```python
from build123d import *

# Parameters (mm, degrees)
SKETCH1_W                                           = 28
SKETCH1_H                                           = 84
BOSS_EXTRUDE2_DEPTH                                 = 15
SKETCH7_W                                           = 54
SKETCH7_H                                           = 12
CUT_EXTRUDE2_DEPTH                                  = 1
CUT_EXTRUDE2_DEPTH_BACK                             = 29
SKETCH6_W                                           = 20
SKETCH6_H                                           = 40.4
CUT_EXTRUDE1_DEPTH                                  = 16
SKETCH8_W                                           = 28
SKETCH8_H                                           = 5
CUT_EXTRUDE3_DEPTH                                  = 7
SKETCH9_R                                           = 1.45
CUT_EXTRUDE4_DEPTH                                  = 6
SKETCH11_R                                          = 4
CUT_EXTRUDE5_DEPTH                                  = 1
CUT_EXTRUDE5_DEPTH_BACK                             = 29
SKETCH12_R                                          = 1.5
CUT_EXTRUDE6_DEPTH                                  = 8
SKETCH13_R                                          = 1.5
CUT_EXTRUDE7_DEPTH                                  = 16
BOSS_EXTRUDE3_DEPTH                                 = 20
CUT_EXTRUDE10_DEPTH                                 = 25
CBORE_FOR_M3_HEX_SOCKET_HEAD_CAP_SCREW1_D           = 3.2
CBORE_FOR_M3_HEX_SOCKET_HEAD_CAP_SCREW1_CBORE_D     = 6.5
CBORE_FOR_M3_HEX_SOCKET_HEAD_CAP_SCREW1_CBORE_DEPTH = 3.4


with BuildPart() as part:
    # Sketch1 → Boss-Extrude2 (new body)
    with BuildSketch(Plane(origin=(0, 0, 0), x_dir=(1, 0, 0), z_dir=(0, 1, 0))):
        with Locations((14, 42)):
            Rectangle(SKETCH1_W, SKETCH1_H)
    extrude(amount=BOSS_EXTRUDE2_DEPTH)

    # Sketch7 → Cut-Extrude2 (cut, two sides)
    with BuildSketch(Plane(origin=(28, 0, 0), x_dir=(0, 0, -1), z_dir=(1, 0, 0))) as cut_extrude2_sk:
        with Locations((42, 6)):
            Rectangle(SKETCH7_W, SKETCH7_H)
    extrude(amount=CUT_EXTRUDE2_DEPTH, mode=Mode.SUBTRACT)
    extrude(cut_extrude2_sk.sketch, amount=-CUT_EXTRUDE2_DEPTH_BACK, mode=Mode.SUBTRACT)

    # Sketch6 → Cut-Extrude1 (cut, through all)
    with BuildSketch(Plane(origin=(0, 15, 0), x_dir=(1, 0, 0), z_dir=(0, 1, 0))):
        with Locations((14, 38.2)):
            Rectangle(SKETCH6_W, SKETCH6_H)
    extrude(amount=-CUT_EXTRUDE1_DEPTH, mode=Mode.SUBTRACT)

    # Sketch8 → Cut-Extrude3 (cut)
    with BuildSketch(Plane.XY):
        with Locations((14, 9.5)):
            Rectangle(SKETCH8_W, SKETCH8_H)
    extrude(amount=-CUT_EXTRUDE3_DEPTH, mode=Mode.SUBTRACT)

    # Sketch9 → Cut-Extrude4 (cut)
    with BuildSketch(Plane(origin=(0, 15, 0), x_dir=(1, 0, 0), z_dir=(0, 1, 0))):
        with Locations((7.5, 13.5)):
            Circle(SKETCH9_R)
        with Locations((20.5, 13.5)):
            Circle(SKETCH9_R)
        with Locations((7.5, 62.9)):
            Circle(SKETCH9_R)
        with Locations((20.5, 62.9)):
            Circle(SKETCH9_R)
    extrude(amount=-CUT_EXTRUDE4_DEPTH, mode=Mode.SUBTRACT)

    # Sketch11 → Cut-Extrude5 (cut, two sides)
    with BuildSketch(Plane.ZY) as cut_extrude5_sk:
        with Locations((-10, 1.5)):
            Circle(SKETCH11_R)
        with Locations((-74, 1.5)):
            Circle(SKETCH11_R)
    extrude(amount=CUT_EXTRUDE5_DEPTH, mode=Mode.SUBTRACT)
    extrude(cut_extrude5_sk.sketch, amount=-CUT_EXTRUDE5_DEPTH_BACK, mode=Mode.SUBTRACT)

    # Sketch12 → Cut-Extrude6 (cut)
    with BuildSketch(Plane.XZ):
        with Locations((4, -3.5)):
            Circle(SKETCH12_R)
        with Locations((24, -3.5)):
            Circle(SKETCH12_R)
    extrude(amount=-CUT_EXTRUDE6_DEPTH, mode=Mode.SUBTRACT)

    # Sketch13 → Cut-Extrude7 (cut, through all)
    with BuildSketch(Plane.XZ):
        with Locations((4, -80.5)):
            Circle(SKETCH13_R)
        with Locations((24, -80.5)):
            Circle(SKETCH13_R)
    extrude(amount=-CUT_EXTRUDE7_DEPTH, mode=Mode.SUBTRACT)

    # Sketch15 → Boss-Extrude3 (add)
    with BuildSketch(Plane(origin=(0, 0, -84), x_dir=(-1, 0, 0), z_dir=(0, 0, -1))):
        with BuildLine():
            Line((-28, 15), (0, 15))
            Line((0, 15), (0, 8.75))
            Line((0, 8.75), (-10.200328962, 8.75))
            ThreePointArc((-10.200328962, 8.75), (-15.594420664, 11.168490527), (-17.506165925, 5.574694698))
            Line((-17.506165925, 5.574694698), (-10.466462197, 5.625403884))
            ThreePointArc((-10.466462197, 5.625403884), (-10.271009725, 6.05271581), (-10.127016654, 6.5))
            Line((-10.127016654, 6.5), (0, 6.5))
            Line((0, 6.5), (0, 0))
            Line((0, 0), (-28, 0))
            Line((-28, 0), (-28, 15))
        make_face()
    extrude(amount=BOSS_EXTRUDE3_DEPTH)

    # Sketch17 → Cut-Extrude10 (cut)
    with BuildSketch(Plane(origin=(0, 0, -104), x_dir=(-1, 0, 0), z_dir=(0, 0, -1))):
        with BuildLine():
            Line((0, 8.75), (-10.200328962, 8.75))
            ThreePointArc((-10.200328962, 8.75), (-15.594420664, 11.168490527), (-17.506165925, 5.574694698))
            Line((-17.506165925, 5.574694698), (-10.466462197, 5.625403884))
            ThreePointArc((-10.466462197, 5.625403884), (-10.271009725, 6.05271581), (-10.127016654, 6.5))
            Line((-10.127016654, 6.5), (0, 6.5))
            Line((0, 6.5), (0, 8.75))
        make_face()
    extrude(amount=-CUT_EXTRUDE10_DEPTH, mode=Mode.SUBTRACT)

    # CBORE for M3 Hex Socket Head Cap Screw1 (through all)
    with Locations(Plane(origin=(7.226315369, 0, -88), x_dir=(0, 0, -1), z_dir=(0, -1, 0))):
        with Locations((0, 0), (10, 0)):
            CounterBoreHole(CBORE_FOR_M3_HEX_SOCKET_HEAD_CAP_SCREW1_D / 2, CBORE_FOR_M3_HEX_SOCKET_HEAD_CAP_SCREW1_CBORE_D / 2, CBORE_FOR_M3_HEX_SOCKET_HEAD_CAP_SCREW1_CBORE_DEPTH)


solid = part.part
```
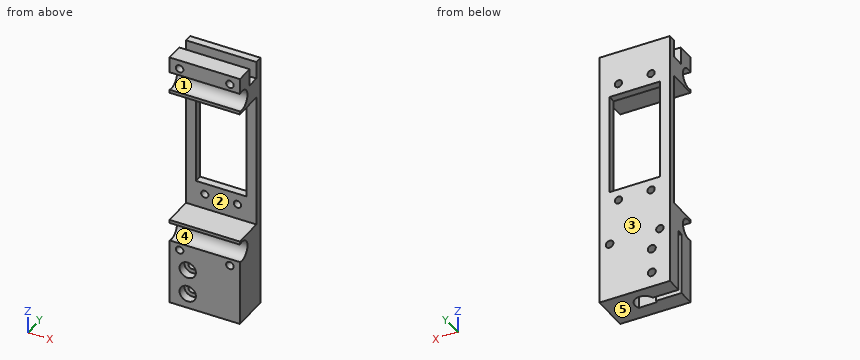
The model under review builds one solid part; all positions refer to its coordinate system, in mm. Face numbers are marked on the shaded views. A direction names the side the tool comes from. Coordinates: 2 decimals unless noted, no trailing zeros. Write each loop counter-clockwise with the first axis right and the second up, starting at its lowest first coordinate (ties: lowest second). Pieces come first, ordered by that corner, then holes. Notation, with made-up numbers: (72.25, -6) -> (121.25, -6) arc R12 ccw to (121.25, 15) -> close; hole circle Ø11 at (59.25, 35.5). An arc over 180 degrees is marked (long way). One line per item, written item: value. Start each with the question number.
Q1. Add section A-A, the plane y = 1. Count the separate pieces of the cut face and the enclosed holes in it, then the cut area to 3 significant figures.
Q2. For the marked faces 1 and 2, list the 3-axis set-ups (+Z, -Z, +X, -X, +Y, -Y) from which the entire face can be reached by the end or side of a thin tool; tool diameter is ignored.
Q3. Add section C-C, the plane x = 20.5. Give the boundary of the cut face in (y, z), then the cut area to 3 significant figures.
Q4. The part is to be moulded in two halves that separate along Z. For the marked faces 3, 4 and 5, say which applies: +Z half, -Z half, draft (parallel to the pull), parting line (faces both ways), or undercut.
Q5. Clearance check with flat-ended pins moving along their axes: P1, Ø5, axis at x = 7, z = -98, coming from the -Y side; P2, Ø1.7, axis at x = 7.5, z = -13.5, coming from the +Y side; P3, Ø3.5, axis at x = 20.5, z = -13.5, coming from the -Y side; P4, Ø12, axis at x = 3.5, z = -54, coming from the -Y side. State where each tip first meets the part, or that it passes through.
Q6. To check wall thickness, follow probe 1 along X at (y, z) = (10.8, -13.5); probe 2 along Z at (x, y) = (17.25, 1.5); probe 3 along Z at (x, y) = (20.5, 13.2). State the ranges of each line that lie inside material, in increasing order.
Q7. Add section D-D, the plane x = 14. Give the boundary of the cut face in (y, z).
Q8. Add section B-B, the plane z = -62.9. Give the boundary of the cut face in (x, y).
Response:
1. separate pieces: 4
1. enclosed holes: 6
1. area: 861 mm²
2. face 1: +X, -X
2. face 2: +X, -X, -Y
3. outline: (0, -104) -> (15, -104) -> (15, -64.35) -> (12, -64.35) -> (12, -69) -> (0, -69) -> (0, -70.29) arc R4 cw (long way) to (0, -77.71) -> close; (0, -15) -> (12, -15) -> (12, -18) -> (15, -18) -> (15, -14.95) -> (9, -14.95) -> (9, -12.05) -> (15, -12.05) -> (15, 0) -> (12, 0) -> (12, -7) -> (7, -7) -> (7, 0) -> (0, 0) -> (0, -6.29) arc R4 cw (long way) to (0, -13.71) -> close; (12, -61.45) -> (15, -61.45) -> (15, -58.4) -> (12, -58.4) -> close
3. area: 656 mm²
4. face 3: draft
4. face 4: undercut
4. face 5: -Z half
5. P1: y = 3.4
5. P2: y = 9
5. P3: y = 0
5. P4: y = 12
6. probe 1: 0 to 6.05, 8.95 to 19.05, 21.95 to 28
6. probe 2: -104 to -78, -70 to -69, -15 to -14, -6 to 0
6. probe 3: -104 to -64.35, -61.45 to -58.4, -18 to -14.95, -12.05 to 0
7. outline: (0, -104) -> (5.6, -104) -> (5.6, -79) -> (11.5, -79) -> (11.5, -104) -> (15, -104) -> (15, -58.4) -> (12, -58.4) -> (12, -69) -> (0, -69) -> (0, -70.29) arc R4 cw (long way) to (0, -77.71) -> close; (0, -15) -> (12, -15) -> (12, -18) -> (15, -18) -> (15, 0) -> (12, 0) -> (12, -7) -> (7, -7) -> (7, 0) -> (0, 0) -> (0, -6.29) arc R4 cw (long way) to (0, -13.71) -> close
8. outline: (0, 12) -> (6.05, 12) -> (6.05, 15) -> (0, 15) -> close; (8.95, 12) -> (19.05, 12) -> (19.05, 15) -> (8.95, 15) -> close; (21.95, 12) -> (28, 12) -> (28, 15) -> (21.95, 15) -> close
